```python
from build123d import *

# Parameters (mm, degrees)
SKETCH_1_W          = 36.5
SKETCH_1_H          = 36.5
EXTRUDE_1_DEPTH     = 5
SKETCH_2_R          = 15
EXTRUDE_2_DEPTH     = 7.5
SKETCH_3_R          = 13.5
EXTRUDE_3_DEPTH     = 5
SKETCH_4_R          = 1.6
CUT_EXTRUDE_1_DEPTH = 29.677081441
FILLET_1_R          = 3


with BuildPart() as part:
    # 草图1 → 凸台-拉伸1 (new body)
    with BuildSketch(Plane.XY):
        Rectangle(SKETCH_1_W, SKETCH_1_H)
    extrude(amount=EXTRUDE_1_DEPTH)

    # 草图2 → 凸台-拉伸2 (add)
    with BuildSketch(Plane.XY.offset(5)):
        Circle(SKETCH_2_R)
    extrude(amount=EXTRUDE_2_DEPTH)

    # 草图3 → 凸台-拉伸3 (add)
    with BuildSketch(Plane(origin=(0, 0, 0), x_dir=(-1, 0, 0), z_dir=(0, 0, -1))):
        with Locations(Location((0, 0, 0), (0, 0, 180))):
            Circle(SKETCH_3_R)
    extrude(amount=EXTRUDE_3_DEPTH)

    # 草图4 → 切除-拉伸1 (cut, through all)
    with BuildSketch(Plane(origin=(0, 0, 0), x_dir=(-1, 0, 0), z_dir=(0, 0, -1))):
        with Locations((-15, 15)):
            Circle(SKETCH_4_R)
        with Locations(Location((-15, -15, 0), (0, 0, 180))):
            Circle(SKETCH_4_R)
        with Locations((15, -15)):
            Circle(SKETCH_4_R)
        with Locations(Location((15, 15, 0), (0, 0, 180))):
            Circle(SKETCH_4_R)
    extrude(amount=-CUT_EXTRUDE_1_DEPTH, mode=Mode.SUBTRACT)

    # 圆角1
    fillet_1_edges = [part.edges().sort_by_distance(p)[0] for p in [
        (-18.25, 18.25, 2.5),
        (18.25, 18.25, 2.5),
        (18.25, -18.25, 2.5),
        (-18.25, -18.25, 2.5),
    ]]
    fillet(fillet_1_edges, radius=FILLET_1_R)


solid = part.part
```
Work out the finished part from the listing and answer in its coordinate system (mm). A direction names the side the tool comes from. Give positions to 0.01 mm unless a question says otherwise; leave off trailing zeros. Write each loop counter-clockwise with the first axis right and the second up, starting at its lowest first coordinate (ties: lowest second). Pieces come first, ordered by that corner, then holes. Notation, with made-up numbers: (34.25, -6) - (72.25, -6) arc R16 cw to (72.25, 2) - close; hole circle Ø5 at (36, 71). An arc over 180 degrees is marked (long way). Use one line per item in the form item = value.
1. For faces 1 (the face through (-16, 0, 5)), 2 (the face through (-8, 12, 0)), 3 (the face through (-17.39, 17.35, 2.54)), determine the directions among +Z, -Z, +X, -X, +Y, -Y from which every point of the face is accessible in a straight line to the end or side of a thin tool.
Filled in:
face_1 = +Z
face_2 = -Z
face_3 = +Z, -Z, -X, +Y
2. A cutting plane is placed at D-D (z = -0.5). Write down the section's boundary in (x, y).
Filled in:
outline = circle Ø27 at (0, 0)
3. A cutting plane is placed at B-B (x = 0). Write down the section's boundary in (y, z).
Filled in:
outline = (-18.25, 0) - (-13.5, 0) - (-13.5, -5) - (13.5, -5) - (13.5, 0) - (18.25, 0) - (18.25, 5) - (15, 5) - (15, 12.5) - (-15, 12.5) - (-15, 5) - (-18.25, 5) - close
4. Consider L1, parallel to Y at x = 15, z = 1.4; L2, parallel to Y at x = 15.5, z = 0.25; L3, parallel to Z at x = 16.5, y = -0.5. Determine where each line is inside the solid, lowest interval first.
Filled in:
L1 = -18.25 to -16.6, -13.4 to 13.4, 16.6 to 18.25
L2 = -18.24 to -16.52, -13.48 to 13.48, 16.52 to 18.24
L3 = 0 to 5
5. Each of these flat-tipped pins is pushed along its axis until it touches: pin 1 Ø6 at (y, z) = (-0.5, 8.5) entering from +X; pin 2 Ø10 at (x, z) = (9, 10.5) entering from -Y; pin 3 Ø5 at (x, y) = (15, 15) entering from +Z. Where does it stop, or does it pass through?
Filled in:
pin_1 = 15
pin_2 = -14.46
pin_3 = 5
6. A cutting plane is placed at A-A (z = 2.5). Write down the section's boundary in (x, y), and give its area (3 significant figures).
Filled in:
outline = (-18.25, -15.25) arc R3 ccw to (-15.25, -18.25) - (15.25, -18.25) arc R3 ccw to (18.25, -15.25) - (18.25, 15.25) arc R3 ccw to (15.25, 18.25) - (-15.25, 18.25) arc R3 ccw to (-18.25, 15.25) - close; hole circle Ø3.2 at (-15, -15); hole circle Ø3.2 at (-15, 15); hole circle Ø3.2 at (15, -15); hole circle Ø3.2 at (15, 15)
area = 1,290 mm^2
